```python
from build123d import *

# Parameters (mm, degrees)
F1_DEPTH    = 6.35
F0_W        = 3.175
F0_H        = 10.795
F2_DEPTH    = 44.45
F3_D        = 15.875
F5_D        = 6.35
F6_DEPTH    = 12.7
F7_T1_DEPTH = 14.2875
F9_DEPTH    = 21.59


# Not quite as in the source:
# - a fillet or chamfer that OpenCascade refuses, or shapes differently, is made with other operations: its cross-section is extruded or revolved along the edge and cut away or added


with BuildPart() as f1:
    # F0 (on Top) → F1 (new body)
    with BuildSketch(Plane.XY):
        with BuildLine():
            Line((22.86, 0), (16.1698598669, 0))
            ThreePointArc((16.1698598669, 0), (29.0375893482, -0.3012781979), (35.56, 10.795))
            ThreePointArc((35.56, 10.795), (29.0375893482, 21.8912781979), (16.1698598669, 21.59))
            Line((16.1698598669, 21.59), (22.86, 21.59))
            Line((22.86, 21.59), (22.86, 0))
        make_face()
        with BuildLine():
            ThreePointArc((16.1698598669, 21.59), (10.16, 10.795), (16.1698598669, 0))
            Line((16.1698598669, 0), (22.86, 0))
            Line((22.86, 0), (22.86, 21.59))
            Line((22.86, 21.59), (16.1698598669, 21.59))
        make_face()
        with BuildLine():
            Line((6.35, 10.795), (6.35, 0))
            Line((6.35, 0), (16.1698598669, 0))
            ThreePointArc((16.1698598669, 0), (10.16, 10.795), (16.1698598669, 21.59))
            Line((16.1698598669, 21.59), (6.35, 21.59))
            Line((6.35, 21.59), (6.35, 10.795))
        make_face()
    extrude(amount=F1_DEPTH)

    # F0 (on Top) → F2 (join)
    with BuildSketch(Plane.XY):
        with Locations((1.5875, 5.3975)):
            Rectangle(F0_W, F0_H)
        with Locations((4.7625, 5.3975)):
            Rectangle(F0_W, F0_H)
        with Locations((4.7625, 16.1925)):
            Rectangle(F0_W, F0_H)
        with Locations((1.5875, 16.1925)):
            Rectangle(F0_W, F0_H)
    extrude(amount=F2_DEPTH)

    # F3 (through all)
    with Locations(Plane(origin=(0, 0, 0), x_dir=(1, 0, 0), z_dir=(0, 0, -1))):
        with Locations((22.86, -10.795)):
            Hole(F3_D / 2)

    # F5 (through all)
    with Locations(Plane.YZ.offset(6.35)):
        with Locations((10.795, 34.925)):
            Hole(F5_D / 2)

    # F4 (on face) → F6 (join)
    with BuildSketch(Plane.YZ.offset(6.35)):
        Polygon((10.795, 12.7), (10.795, 19.05), (7.747, 19.05), (7.747, 6.35), (10.795, 6.35), align=None)
        Polygon((13.843, 19.05), (10.795, 19.05), (10.795, 12.7), (10.795, 6.35), (13.843, 6.35), align=None)
    extrude(amount=-F6_DEPTH)

    # F7: fillet of radius 3.175 on 2 edges, made by hand

    # F7_s2 → F7_t1 (cut)
    with BuildSketch(Plane.YZ.offset(-14.2875)):
        with BuildLine():
            ThreePointArc((10.922, 6.35), (8.6769359697, 7.2799359697), (7.747, 9.525))
            Line((7.747, 9.525), (7.747, 6.35))
            Line((7.747, 6.35), (10.922, 6.35))
        make_face()
        with BuildLine():
            ThreePointArc((13.843, 9.525), (12.9130640303, 7.2799359697), (10.668, 6.35))
            Line((10.668, 6.35), (13.843, 6.35))
            Line((13.843, 6.35), (13.843, 9.525))
        make_face()
    extrude(amount=F7_T1_DEPTH, mode=Mode.SUBTRACT)

    # F8 (on face) → F9 (join)
    with BuildSketch(Plane.XZ):
        Polygon((11.2599299335, 6.35), (6.35, 12.7), (6.35, 6.35), align=None)
    extrude(amount=-F9_DEPTH)


solid = f1.part
```
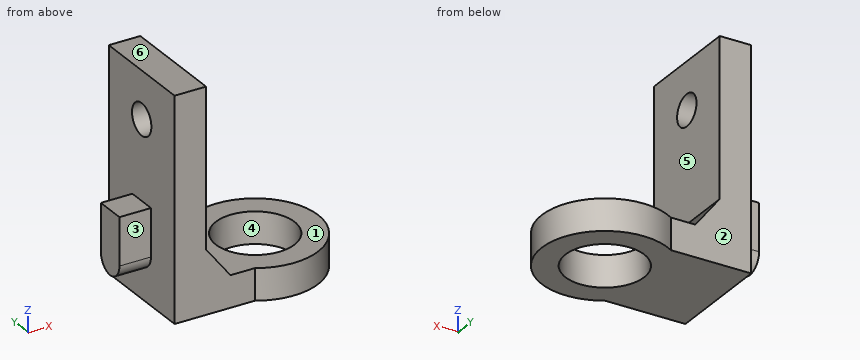
Geometry check sheet. Reference: the model listing, model coordinates, mm. Face numbers are marked on the shaded views. A direction names the side the tool comes from. Give positions to 0.01 mm unless a question says otherwise; leave off trailing zeros. Order: outer loops, then holes, each group sorted by start corner. A loop starts at its lowest first (then second) coordinate and runs counter-clockwise, first axis right, second up. Notation, with made-up numbers: (40, 34.5) - (44, 34.5) arc R18 ccw to (44, 53.5) - close; hole circle Ø10 at (-18.5, 50.25). An arc over 180 degrees is marked (long way). Answer in a Markdown table with one row per item. Add a question column.
Q1. Material ranges on probe 1 along Z at (x, y) = (14.5, 2.75); probe 2 along Z at (x, y) = (1.5, 11), recorded low to high. Write a range as from..to.
Q2. Gauge pin test, flat ends, axial feed: pin 1 (3 mm diameter, centred on x = -2.5, z = 14, fed in from -Y); pin 2 (4 mm diameter, centred on y = 12.5, z = 29, fed in from +X); pin 3 (6.5 mm diameter, centred on x = -2, y = 10.5, fed in from +Z); pin 4 (2 mm diameter, centred on x = 9, y = 9, fed in from +Z). Record the tip position at first contact, or that the pin passes through.
Q3. Cross-section at B-B, the plane y = 13. Enter the section's corners in (x, z).
Q4. Cross-section at D-D, the plane z = 35.5. Enter the section's corners in (x, y), then the cut area to 3 significant figures.
Q5. Mould release check, pull along X, two halves, no side actions. Record for the marked faces 4, 5 and 6: pulls with the +X half, pulls with the -X half, needs draft (parallel to the pull), parting line crosses it, or undercut.
Q6. Cross-section at C-C, the plane z = 4. Enter the section's corners in (x, y) (1 decimal).
Q7. Tool access check on the marked faces 1, 2 and 3. Record the directions out of +Z, -Z, +X, -X, +Y, -Y that give a thin tool (end or side, any length) a straight path to the whole face; none if there is none.
Check values:
| question | item | result |
|---|---|---|
| 1 | probe 1 | z = 0..6.35 |
| 1 | probe 2 | z = 0..31.76, 38.09..44.45 |
| 2 | pin 1 | stops at y = 7.75 |
| 2 | pin 2 | stops at x = 6.35 |
| 2 | pin 3 | stops at z = 44.45 |
| 2 | pin 4 | stops at z = 10.57 |
| 3 | outline | (-6.35, 7.37) - (0, 7.37) - (0, 0) - (15.23, 0) - (15.23, 6.35) - (11.26, 6.35) - (6.35, 12.7) - (6.35, 32.64) - (0, 32.64) - (0, 19.05) - (-6.35, 19.05) - close; (0, 37.21) - (6.35, 37.21) - (6.35, 44.45) - (0, 44.45) - close; (30.49, 0) - (35.37, 0) - (35.37, 6.35) - (30.49, 6.35) - close |
| 4 | outline | (0, 0) - (6.35, 0) - (6.35, 7.67) - (0, 7.67) - close; (0, 13.92) - (6.35, 13.92) - (6.35, 21.59) - (0, 21.59) - close |
| 4 | area | 97.4 mm^2 |
| 5 | face 4 | undercut |
| 5 | face 5 | pulls with the +X half |
| 5 | face 6 | needs draft |
| 6 | outline | (0, 0) - (16.2, 0) arc R12.7 ccw (long way) to (16.2, 21.6) - (0, 21.6) - close; hole circle Ø15.9 at (22.9, 10.8) |
| 7 | face 1 | +Z, +X, +Y, -Y |
| 7 | face 2 | +Z, -Z, -X, +Y |
| 7 | face 3 | +Z, -Z, -X, -Y |
